from build123d import *

# Parameters (mm, degrees)
SKETCH1_R            = 6
BODY_DEPTH           = 19
SKETCH2_R            = 1.5
HOLES_DEPTH          = 7
HOLES_DEPTH_BACK     = 7
F_1X_45_CHAMFER_SIZE = 0.5


with BuildPart() as part:
    # Sketch1 → Body (new body, symmetric)
    with BuildSketch(Plane.XY):
        Circle(SKETCH1_R)
    extrude(amount=BODY_DEPTH, both=True)

    # Sketch2 → Holes (cut, two sides)
    with BuildSketch(Plane(origin=(0, 0, 0), x_dir=(0, 0, -1), z_dir=(1, 0, 0))) as holes_sk:
        with Locations((-14, 0)):
            Circle(SKETCH2_R)
        with Locations((14, 0)):
            Circle(SKETCH2_R)
    extrude(amount=HOLES_DEPTH, mode=Mode.SUBTRACT)
    extrude(holes_sk.sketch, amount=-HOLES_DEPTH_BACK, mode=Mode.SUBTRACT)

    # 1x 45 Chamfer
    f_1x_45_chamfer_edges = [part.edges().sort_by_distance(p)[0] for p in [
        (-6, 0, -19),
        (-6, 0, 19),
    ]]
    chamfer(f_1x_45_chamfer_edges, length=F_1X_45_CHAMFER_SIZE)


solid = part.part
Work out the finished part from the listing and answer in its coordinate system (mm). Give positions to 0.01 mm unless a question says otherwise; leave off trailing zeros. Write each loop counter-clockwise with the first axis right and the second up, starting at its lowest first coordinate (ties: lowest second). Pieces come first, ordered by that corner, then holes. Notation, with made-up numbers: (-10.75, 69) - (12.25, 69) arc R10 ccw to (12.25, 73) - close; hole circle Ø1 at (40.25, 8.5). An arc over 180 degrees is marked (long way). One line per item, written item: value. Start each with the question number.
1. Consider probe 1 along Z at (x, y) = (2.75, 0); probe 2 along Z at (x, y) = (4.25, 1); probe 3 along Y at (x, z) = (3.5, 14). Determine where each line is inside the solid, lowest interval first.
2. Find section C-C (x = -4.5). State how many separate pieces and enclosed holes the cut face has, then the cut area to 3 significant figures.
3. Find section B-B (z = 14). Write down the section's boundary in (x, y), then the cut area to 3 significant figures.
4. Find section A-A (y = 0). Write down the section's boundary in (x, z).
5. Given pin 1 (2.5 mm diameter, centred on y = 0, z = 14, fed in from -X); pin 2 (1 mm diameter, centred on y = -0.5, z = 9.5, fed in from -X); pin 3 (2 mm diameter, centred on y = -3.5, z = -1, fed in from -X); pin 4 (1 mm diameter, centred on x = -4.5, z = 4, fed in from -Y), each flat-ended and moving along its own axis, determine where each tip first touches the part or whether it passes through.
Geometry results:
1. probe 1: -19 to -15.5, -12.5 to 12.5, 15.5 to 19
1. probe 2: -19 to -15.12, -12.88 to 12.88, 15.12 to 19
1. probe 3: -4.87 to -1.5, 1.5 to 4.87
2. separate pieces: 1
2. enclosed holes: 2
2. area: 287 mm2
3. outline: (-5.81, -1.5) arc R6 ccw to (5.81, -1.5) - close; (-5.81, 1.5) - (5.81, 1.5) arc R6 ccw to start
3. area: 77.5 mm2
4. outline: (-6, -18.5) - (-5.5, -19) - (5.5, -19) - (6, -18.5) - (6, -15.5) - (-6, -15.5) - close; (-6, -12.5) - (6, -12.5) - (6, 12.5) - (-6, 12.5) - close; (-6, 15.5) - (6, 15.5) - (6, 18.5) - (5.5, 19) - (-5.5, 19) - (-6, 18.5) - close
5. pin 1: through
5. pin 2: x = -6
5. pin 3: x = -5.45
5. pin 4: y = -4.47
